```python
from build123d import *

# Parameters (mm, degrees)
BOSS_EXTRUDE3_DEPTH      = 10
BOSS_EXTRUDE3_DEPTH_BACK = 5
SKETCH3_R                = 6
SKETCH3_R_2              = 3.3
SKETCH10_R               = 12.775
SKETCH10_R_2             = 3.65
SKETCH10_R_3             = 2.1
BOSS_EXTRUDE5_DEPTH      = 2
SKETCH11_R               = 11.275
SKETCH11_R_2             = 6.775
BOSS_EXTRUDE6_DEPTH      = 0.8
SKETCH12_R               = 1.25
CUT_EXTRUDE2_DEPTH       = 2.75
FILLET3_R                = 1
SKETCH13_R               = 12.775
SKETCH13_R_2             = 11.275
BOSS_EXTRUDE7_DEPTH      = 10
SKETCH14_R               = 11.7
CUT_EXTRUDE3_DEPTH       = 9.2
CUT_EXTRUDE5_DEPTH       = 16
SKETCH16_R               = 4.5
CUT_EXTRUDE6_DEPTH       = 14


with BuildPart() as part:
    # Sketch3 → Boss-Extrude3 (new, two sides: drawn at the far end of the back side and taken through both)
    with BuildSketch(Plane(origin=(0, 0, 0), x_dir=(0, 0, -1), z_dir=(1, 0, 0)).offset(-BOSS_EXTRUDE3_DEPTH_BACK)):
        Circle(SKETCH3_R)
        Circle(SKETCH3_R_2, mode=Mode.SUBTRACT)
    extrude(amount=BOSS_EXTRUDE3_DEPTH + BOSS_EXTRUDE3_DEPTH_BACK)

    # Sketch10 → Boss-Extrude5 (add)
    # profile 1 of 2: a face of its own
    with BuildSketch(Plane(origin=(10, 0, 0), x_dir=(0, 0, -1), z_dir=(1, 0, 0))):
        Circle(SKETCH10_R)
        Circle(SKETCH10_R_2, mode=Mode.SUBTRACT)
    # profile 2 of 2: a face of its own
    with BuildSketch(Plane(origin=(10, 0, 0), x_dir=(0, 0, -1), z_dir=(1, 0, 0))):
        Circle(SKETCH10_R_3)
    extrude(amount=-BOSS_EXTRUDE5_DEPTH)


with BuildPart() as boss_extrude5_kept_piece:
    # of the separate pieces the step leaves, the one the design keeps (boss_extrude5_pieces_kept)
    add(part.part.solids().sort_by_distance((0, 0, -6))[0])

    # Sketch11 → Boss-Extrude6 (add)
    with BuildSketch(Plane(origin=(10, 0, 0), x_dir=(0, 0, -1), z_dir=(1, 0, 0))):
        Circle(SKETCH11_R)
        Circle(SKETCH11_R_2, mode=Mode.SUBTRACT)
    extrude(amount=BOSS_EXTRUDE6_DEPTH)

    # Sketch12 → Cut-Extrude2 (cut)
    with BuildSketch(Plane(origin=(10.8, 0, 0), x_dir=(0, 0, -1), z_dir=(1, 0, 0))):
        with BuildLine():
            ThreePointArc((9.330017017, -4.665), (8.705017017, -3.582468245), (7.455017017, -3.582468245))
            Line((7.455017017, -3.582468245), (8.080017017, -4.665))
            Line((8.080017017, -4.665), (6.830017017, -4.665))
            ThreePointArc((6.830017017, -4.665), (8.080017017, -5.915), (9.330017017, -4.665))
        make_face()
        with BuildLine():
            Line((8.080017017, -4.665), (7.455017017, -3.582468245))
            ThreePointArc((7.455017017, -3.582468245), (6.997485263, -4.04), (6.830017017, -4.665))
            Line((6.830017017, -4.665), (8.080017017, -4.665))
        make_face()
        with BuildLine():
            Line((0.625, 8.247468245), (0, 9.33))
            Line((0, 9.33), (-0.625, 8.247468245))
            ThreePointArc((-0.625, 8.247468245), (0, 8.08), (0.625, 8.247468245))
        make_face()
        with BuildLine():
            Line((-0.625, 8.247468245), (0, 9.33))
            Line((0, 9.33), (0.625, 8.247468245))
            ThreePointArc((0.625, 8.247468245), (1.082531755, 8.705), (1.25, 9.33))
            ThreePointArc((1.25, 9.33), (-0.625, 10.412531755), (-0.625, 8.247468245))
        make_face()
        with Locations((-8.080017017, -4.665)):
            Circle(SKETCH12_R)
    extrude(amount=-CUT_EXTRUDE2_DEPTH, mode=Mode.SUBTRACT)

    # Fillet3
    fillet3_edges = [boss_extrude5_kept_piece.edges().sort_by_distance(p)[0] for p in [
        (8, 0, 12.775),
    ]]
    fillet(fillet3_edges, radius=FILLET3_R)

    # Sketch13 → Boss-Extrude7 (add)
    with BuildSketch(Plane(origin=(10, 0, 0), x_dir=(0, 0, -1), z_dir=(1, 0, 0))):
        Circle(SKETCH13_R)
        Circle(SKETCH13_R_2, mode=Mode.SUBTRACT)
    extrude(amount=BOSS_EXTRUDE7_DEPTH)

    # Sketch14 → Cut-Extrude3 (cut)
    with BuildSketch(Plane(origin=(20, 0, 0), x_dir=(0, 0, -1), z_dir=(1, 0, 0))):
        Circle(SKETCH14_R)
    extrude(amount=-CUT_EXTRUDE3_DEPTH, mode=Mode.SUBTRACT)

    # Sketch15 → Cut-Extrude5 (cut)
    with BuildSketch(Plane(origin=(0, 0, 0), x_dir=(1, 0, 0), z_dir=(0, 1, 0))):
        with BuildLine():
            Line((15.430071931, 3.675), (20, 3.675))
            Line((20, 3.675), (20, 11.775))
            Line((20, 11.775), (15.430071931, 11.775))
            ThreePointArc((15.430071931, 11.775), (11.380071931, 7.725), (15.430071931, 3.675))
        make_face()
    extrude(amount=CUT_EXTRUDE5_DEPTH, mode=Mode.SUBTRACT)

    # Sketch16 → Cut-Extrude6 (cut)
    with BuildSketch(Plane.ZY.offset(5)):
        Circle(SKETCH16_R)
    extrude(amount=-CUT_EXTRUDE6_DEPTH, mode=Mode.SUBTRACT)


solid = boss_extrude5_kept_piece.part
```
Geometry check sheet. Reference: the model listing, model coordinates, mm. A direction names the side the tool comes from. Coordinates: 2 decimals unless noted, no trailing zeros. Order: outer loops, then holes, each group sorted by start corner. A loop starts at its lowest first (then second) coordinate and runs counter-clockwise, first axis right, second up. Notation, with made-up numbers: M 65.5,70 L 100.5,70 A17 cw 100.5,75 Z; hole C 32,78.25 d2. An arc over 180 degrees is marked long. One line per question, with ' | ' between items. Start each with the question number.
Item 1: Draft check along Z on faces 1 (the flat face through (8, -5, -5)), 2 (the cylindrical face through (9.49, 2.23, 2.43)), 3 (the cylindrical face through (1, 0, 6)), 4 (the flat face through (18, 12, -3.675)). Enter one of: pulls with the +Z half, pulls with the -Z half, needs draft (parallel to the pull), parting line crosses it, or undercut.
Item 2: Cross-section at C-C on x = 7. Enter the section's corners in (y, z), then the cut area to 3 significant figures.
Item 3: Gauge pin test, flat ends, axial feed: pin 1 (3 mm diameter, centred on x = 5.5, z = 3, fed in from +Y); pin 2 (4.5 mm diameter, centred on y = 2, z = 0.5, fed in from -X); pin 3 (8 mm diameter, centred on x = -2.5, y = 2.5, fed in from -Z). Record the tip position at first contact, or that the pin passes through.
Item 4: Cross-section at B-B on x = 16.25. Enter the section's corners in (y, z) (3 decimals).
Item 5: Material ranges on L1, parallel to Y at x = 9.7, z = 0 (3 decimals); L2, parallel to Y at x = 14.75, z = 0 (3 decimals); L3, parallel to Y at x = 8.65, z = 0, recorded low to high. Write a range as [from, to].
Item 6: Set-up check for faces 5 (the flat face through (-5, 4.5, 1.4)), 6 (the cylindrical face through (15.5, -7.1, 9.3)), 7 (the cylindrical face through (1.9, 4.46, -0.59)), 8 (the flat face through (18, 2, -11.775)): record each of +Z, -Z, +X, -X, +Y, -Y from which the full face is reachable in a straight line by a thin tool's end or side.
Findings:
1) face 1: needs draft | face 2: undercut | face 3: parting line crosses it | face 4: pulls with the -Z half
2) outline: C 0,0 d12; hole C 0,0 d9 | area: 49.5 mm²
3) pin 1: stops at y = 5.81 | pin 2: stops at x = 9 | pin 3: stops at z = -6
4) outline: M 0,-11.775 L 0,-11.7 A11.7 cw long 11.108,-3.675 L 12.235,-3.675 A12.775 ccw long 4.955,-11.775 Z
5) L1: y = [-12.775, -3.3], [3.3, 8.08], [10.58, 12.775] | L2: y = [-12.775, -11.7], [11.7, 12.775] | L3: y = [-12.71, -4.5], [4.5, 8.08], [10.58, 12.71]
6) face 5: +Z, -Z, -X, +Y, -Y | face 6: +X | face 7: -X | face 8: +X, +Y
